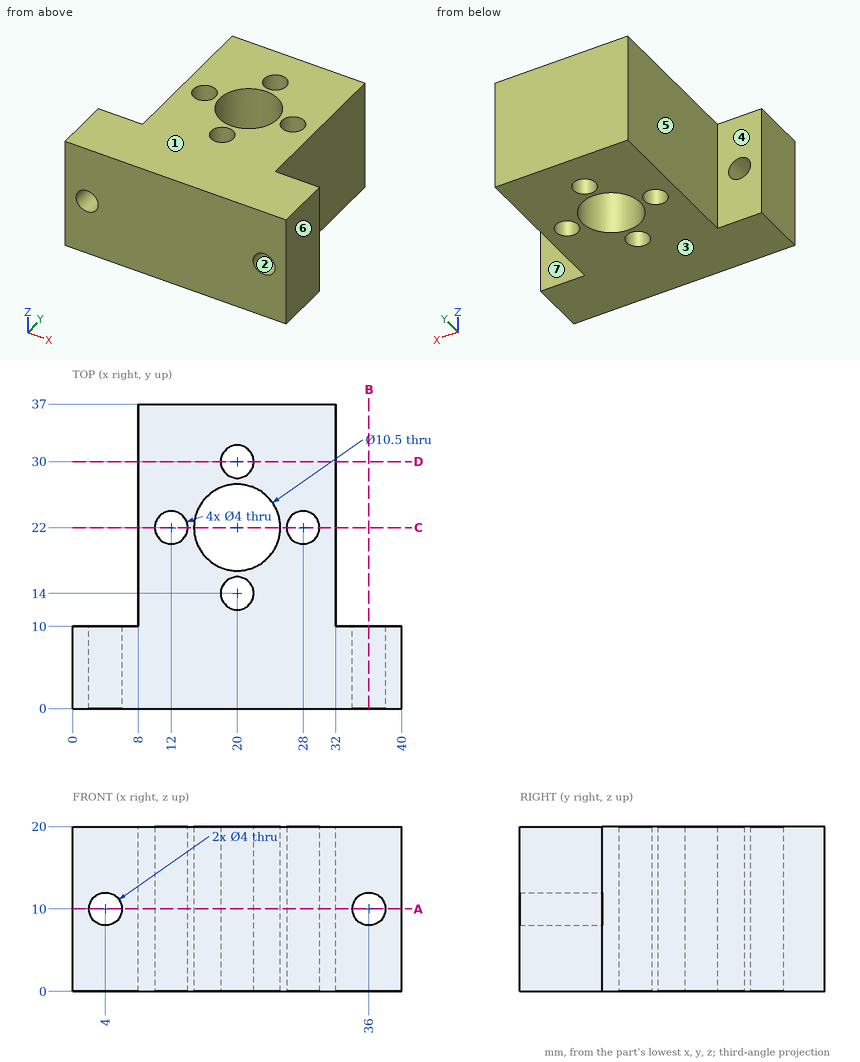
Source: three-view drawing plus pictorial views. Frame: mm from the lowest corner of the part. A direction names the side the tool comes from. Round coordinates to 2 decimals unless told otherwise and drop trailing zeros. Order: outer loops, then holes, each group sorted by start corner. A loop starts at its lowest first (then second) coordinate and runs counter-clockwise, first axis right, second up. Notation, with made-up numbers: M 37,-19.75 L 70,-19.75 A17 ccw 70,-10.75 Z; hole C 59.25,68.25 d5. An arc over 180 degrees is marked long. One line per item, written item: value.
(1) Pull-direction query (Z, two-part tool) for the marked faces 1, 2, 3 and 4; classes: pulls with the +Z half, pulls with the -Z half, needs draft (parallel to the pull), parting line crosses it, or undercut.
Result sheet:
face 1: pulls with the +Z half
face 2: undercut
face 3: pulls with the -Z half
face 4: needs draft
(2) Cut plane B-B (x = 36). Return the cut outline in (y, z), and give its area (3 significant figures).
Result sheet:
outline: M 0,0 L 10,0 L 10,8 L 0,8 Z; M 0,12 L 10,12 L 10,20 L 0,20 Z
area: 160 mm2
(3) Cut plane A-A (z = 10). Return the cut outline in (x, y).
Result sheet:
outline: M 0,0 L 2,0 L 2,10 L 0,10 Z; M 6,0 L 34,0 L 34,10 L 32,10 L 32,37 L 8,37 L 8,10 L 6,10 Z; M 38,0 L 40,0 L 40,10 L 38,10 Z; hole C 12,22 d4; hole C 20,22 d10.5; hole C 20,14 d4; hole C 20,30 d4; hole C 28,22 d4
(4) Cut plane D-D (y = 30). Return the cut outline in (x, z), and give its area (3 significant figures).
Result sheet:
outline: M 8,0 L 18,0 L 18,20 L 8,20 Z; M 22,0 L 32,0 L 32,20 L 22,20 Z
area: 400 mm2
(5) Reachability of the marked faces 5, 6 and 7 from +Z, -Z, +X, -X, +Y, -Y: full face, straight path, thin tool, end or side. Return the list, or none.
Result sheet:
face 5: +Z, -Z, -X, +Y
face 6: +Z, -Z, +X, +Y, -Y
face 7: +Z, -Z, +X, +Y
(6) Line query: probe 1 along Y at (x, z) = (20, 10); probe 2 along Z at (x, y) = (36, 3); probe 3 along Y at (x, z) = (33.5, 19.25). Output: solid intervals per line, ascending. Write a range as [from, to].
Result sheet:
probe 1: [0, 12], [16, 16.75], [27.25, 28], [32, 37]
probe 2: [0, 8], [12, 20]
probe 3: [0, 10]
(7) Cut plane C-C (y = 22). Return the cut outline in (x, z).
Result sheet:
outline: M 8,0 L 10,0 L 10,20 L 8,20 Z; M 14,0 L 14.75,0 L 14.75,20 L 14,20 Z; M 25.25,0 L 26,0 L 26,20 L 25.25,20 Z; M 30,0 L 32,0 L 32,20 L 30,20 Z
(8) Pin query (flat end, axial travel): P1, Ø6, axis at y = 20, z = 3.5, coming from the -X side; P2, Ø5, axis at y = 16.5, z = 14, coming from the +X side; P3, Ø2.5, axis at x = 20, y = 30, coming from the -Z side; P4, Ø6.5, axis at x = 36, z = 10, coming from the +Y side. Return the tip coordinate at first contact, or that it passes through.
Result sheet:
P1: x = 8
P2: x = 32
P3: through
P4: y = 10
